from build123d import *

# Parameters (mm, degrees)
BODY_DEPTH = 0.6


with BuildPart() as part:
    # BodySke → Body (new body)
    with BuildSketch(Plane.XY):
        with BuildLine():
            Line((3.542798702, -3.542798702), (2.874267987, -3.542798702))
            ThreePointArc((2.874267987, -3.542798702), (2.154333999, -3.244592279), (1.856127576, -2.524658291))
            Line((1.856127576, -2.524658291), (1.856127576, -0.523137995))
            ThreePointArc((1.856127576, -0.523137995), (1.884318549, -0.455078967), (1.952377576, -0.426887995))
            Line((1.952377576, -0.426887995), (3.664158868, -0.426887995))
            ThreePointArc((3.664158868, -0.426887995), (3.976794043, -0.270800915), (4.039911091, 0.072885231))
            ThreePointArc((4.039911091, 0.072885231), (2.986408887, 1.865726167), (1.202703544, 2.934623154))
            ThreePointArc((1.202703544, 2.934623154), (0.900072735, 2.901285473), (0.713027436, 2.661054618))
            Line((0.713027436, 2.661054618), (0.498226662, 1.859407216))
            ThreePointArc((0.498226662, 1.859407216), (0, 1.925), (-0.498226662, 1.859407216))
            Line((-0.498226662, 1.859407216), (-0.713027436, 2.661054618))
            ThreePointArc((-0.713027436, 2.661054618), (-0.900072735, 2.901285473), (-1.202703544, 2.934623154))
            ThreePointArc((-1.202703544, 2.934623154), (-2.986408887, 1.865726167), (-4.039911091, 0.072885231))
            ThreePointArc((-4.039911091, 0.072885231), (-3.976794043, -0.270800915), (-3.664158868, -0.426887995))
            Line((-3.664158868, -0.426887995), (-1.952377576, -0.426887995))
            ThreePointArc((-1.952377576, -0.426887995), (-1.884318549, -0.455078967), (-1.856127576, -0.523137995))
            Line((-1.856127576, -0.523137995), (-1.856127576, -2.524658291))
            ThreePointArc((-1.856127576, -2.524658291), (-2.154333999, -3.244592279), (-2.874267987, -3.542798702))
            Line((-2.874267987, -3.542798702), (-3.542798702, -3.542798702))
            ThreePointArc((-3.542798702, -3.542798702), (0, 5.010273973), (3.542798702, -3.542798702))
        make_face()
    extrude(amount=-BODY_DEPTH)


solid = part.part
Here's how the part is built. I have some questions about the finished solid (model axes, mm). A direction names the side the tool comes from. Coordinates: 2 decimals unless noted, no trailing zeros. Write each loop counter-clockwise with the first axis right and the second up, starting at its lowest first coordinate (ties: lowest second). Pieces come first, ordered by that corner, then holes.
1) If we section it at D-D (x = 0): List the corners of the cut face in (y, z) for me (3 decimals), plus the area to 3 significant figures.
Filled in:
outline: (1.925, -0.6) - (5.01, -0.6) - (5.01, 0) - (1.925, 0) - close
area: 1.85 mm2
2) If we section it at B-B (y = -2.75): List the corners of the cut face in (x, z) for me.
Filled in:
outline: (-4.19, -0.6) - (-1.88, -0.6) - (-1.88, 0) - (-4.19, 0) - close; (1.88, -0.6) - (4.19, -0.6) - (4.19, 0) - (1.88, 0) - close
3) If I drill on line 1 (X direction, y = 0, z = -0.15); line 2 (X direction, y = 2.25, z = -0.45); line 3 (X direction, y = 2.5, z = -0.35), over which ranges is the centre line in solid material (lowest first)?
Filled in:
line 1: x = -5.01 to -4.05, 4.05 to 5.01
line 2: x = -4.48 to -2.55, -0.6 to 0.6, 2.55 to 4.48
line 3: x = -4.34 to -2.18, -0.67 to 0.67, 2.18 to 4.34
4) Thinking about a two-plate mould opening in Y: for faces 1 (the face through (0, 3, 0)), 2 (the face through (-2.966, 1.887, -0.296)), 3 (the face through (-0.165, 5.008, -0.296)), 4 (the face through (-2.15, -3.24, -0.3)), which applies, +Y half, -Y half, draft (parallel to the pull), parting line (faces both ways), or undercut?
Filled in:
face 1: draft
face 2: undercut
face 3: parting line
face 4: -Y half
5) If we section it at C-C (y = 2.25): List the corners of the cut face in (x, z) for me, plus the area to 3 significant figures.
Filled in:
outline: (-4.48, -0.6) - (-2.55, -0.6) - (-2.55, 0) - (-4.48, 0) - close; (-0.6, -0.6) - (0.6, -0.6) - (0.6, 0) - (-0.6, 0) - close; (2.55, -0.6) - (4.48, -0.6) - (4.48, 0) - (2.55, 0) - close
area: 3.04 mm2
6) Which directions (+Z, -Z, +X, -X, +Y, -Y) give clear straight access to the entire face, cutting with the end or side of a thin tool? Please do faces 5 (the face through (2.16, -3.25, -0.3)), 6 (the face through (3.01, 1.84, -0.3)), 7 (the face through (0, 3, -0.6)).
Filled in:
face 5: +Z, -Z, -Y
face 6: +Z, -Z
face 7: -Z, +X, -X, +Y, -Y
